Part model, mm, in its own coordinate system. Face numbers are marked on the shaded views. A direction names the side the tool comes from. Round coordinates to 2 decimals unless told otherwise and drop trailing zeros. Loops run counter-clockwise (first coordinate to the right, second up) from the corner with the lowest first, then second, coordinate; pieces in that order, holes last. Notation, with made-up numbers: (50.25, -19.75) -> (78.25, -19.75) arc R25 cw to (78.25, 4.25) -> close; hole circle Ø9 at (45.5, -35.75). An arc over 180 degrees is marked (long way). Answer as CSV lines item,"result".
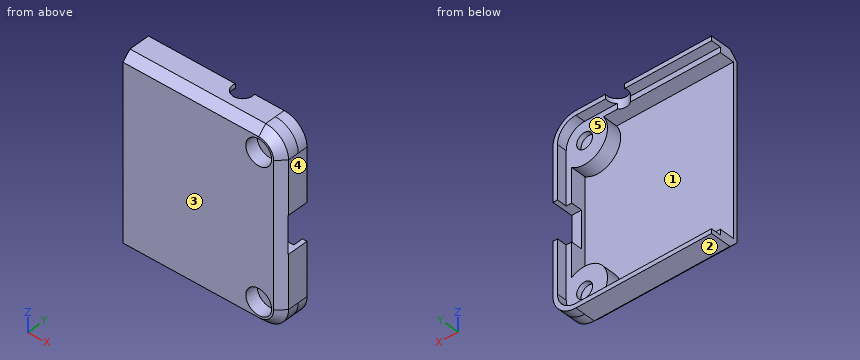
from build123d import *

# Parameters (mm, degrees)
CYLINDER003_R     = 2
CYLINDER003_DEPTH = 10
CYLINDER001_R     = 2
CYLINDER001_DEPTH = 10
SKETCH037_W       = 7.5
SKETCH037_H       = 7.5
EXTRUDE045_DEPTH  = 10
SKETCH032_R       = 2.6
EXTRUDE043_DEPTH  = 0.8
EXTRUDE050_DEPTH  = 3
EXTRUDE051_DEPTH  = 0.8
EXTRUDE038_DEPTH  = 2


with BuildPart() as shutter_cable001:
    # Cylinder003 → Cylinder003 (new body)
    with BuildSketch(Plane(origin=(19.5, 0, 24.5), x_dir=(1, 0, 0), z_dir=(0, 0, 1))):
        Circle(CYLINDER003_R)
    extrude(amount=CYLINDER003_DEPTH)


with BuildPart() as battery_cable:
    # Cylinder001 → Cylinder001 (new body)
    with BuildSketch(Plane(origin=(-70.5, 0, 12), x_dir=(0, 0, 1), z_dir=(-1, 0, 0))):
        Circle(CYLINDER001_R)
    extrude(amount=CYLINDER001_DEPTH)


with BuildPart() as common_sub:
    # Sketch037 → Extrude045 (new body)
    with BuildSketch(Plane.YZ.offset(35)):
        with Locations((0, 12)):
            Rectangle(SKETCH037_W, SKETCH037_H)
    extrude(amount=EXTRUDE045_DEPTH)


with BuildPart() as common_sub_1:
    # Extrude045 placement: moved
    add(common_sub.part.moved(Location((-9.5, 0, 0))))

    # Fusion033: union shutter cable001, battery cable
    add(shutter_cable001.part)
    add(battery_cable.part)


with BuildPart() as sweep_body:
    # Sweep: sweep along a path in Sketch034
    with BuildLine(Plane.XZ.offset(10)) as sweep_path:
        Line((32, 12), (32, 26.4))
        ThreePointArc((32, 26.4), (30.652691, 29.652691), (27.4, 31))
        Line((27.4, 31), (-39.9, 31))
    # Sketch033 → Sweep (sweep)
    with BuildSketch(Plane.YZ):
        Polygon((-5.3, 29.4), (-3.7, 31), (-3.7, 32), (-6, 32), (-6, 29.4), align=None)
    sweep(path=sweep_path.line)


with BuildPart() as fusion:
    # Sketch032 → Extrude043 (new body)
    with BuildSketch(Plane.XZ.offset(10)):
        with Locations((27.4, 26.4)):
            Circle(SKETCH032_R)
    extrude(amount=EXTRUDE043_DEPTH)


with BuildPart() as fusion_1:
    # Extrude043 placement: moved
    add(fusion.part.moved(Location((0, 5.5, 0))))

    # Fusion: union Sweep body
    add(sweep_body.part)


with BuildPart() as screw_hole_bottom002:
    # Sketch003 → Revolve (revolve)
    with BuildSketch(Plane.XY):
        Polygon((1.6, 3), (1.6, 2), (0, 2), (0, 1.8), (2.6, 1.8), (2.6, 0), (4.6, 0), (4.6, 3), align=None)
    revolve(axis=Axis((0, 0, 0), (0, 1, 0)))


with BuildPart() as screw_hole_bottom002_1:
    # Body003 placement: moved
    add(screw_hole_bottom002.part.moved(Location((27.4, -4.5, 26.4))))


with BuildPart() as bottom009:
    # Sketch041 → Extrude050 (new body)
    with BuildSketch(Plane.XZ.offset(10)):
        with BuildLine():
            ThreePointArc((32, 26.4), (30.652691, 29.652691), (27.4, 31))
            Line((27.4, 31), (0.1, 31))
            Line((0.1, 31), (0.1, 29))
            Line((0.1, 29), (27.4, 29))
            ThreePointArc((30, 26.4), (29.238478, 28.238478), (27.4, 29))
            Line((30, 12), (30, 26.4))
            Line((32, 12), (30, 12))
            Line((32, 26.4), (32, 12))
        make_face()
    extrude(amount=EXTRUDE050_DEPTH)


with BuildPart() as bottom009_1:
    # Extrude050 placement: moved
    add(bottom009.part.moved(Location((0, 8.5, 0))))


with BuildPart() as bottom010:
    # Sketch042 → Extrude051 (new body)
    with BuildSketch(Plane.XZ.offset(10)):
        with BuildLine():
            ThreePointArc((32, 26.4), (30.652691, 29.652691), (27.4, 31))
            Line((27.4, 31), (0.1, 31))
            Line((0.1, 31), (0.1, 12))
            Line((0.1, 12), (32, 12))
            Line((32, 26.4), (32, 12))
        make_face()
    extrude(amount=EXTRUDE051_DEPTH)


with BuildPart() as bottom010_1:
    # Extrude051 placement: moved
    add(bottom010.part.moved(Location((0, 5.5, 0))))


with BuildPart() as bottom:
    # Sketch030 → Extrude038 (new body)
    with BuildSketch(Plane.XZ.offset(10)):
        with BuildLine():
            ThreePointArc((32, 26.4), (30.652691, 29.652691), (27.4, 31))
            Line((27.4, 31), (0.1, 31))
            Line((0.1, 31), (0.1, 30.1))
            Line((0.1, 30.1), (27.4, 30.1))
            ThreePointArc((31.1, 26.4), (30.016295, 29.016295), (27.4, 30.1))
            Line((31.1, 12), (31.1, 26.4))
            Line((32, 12), (31.1, 12))
            Line((32, 26.4), (32, 12))
        make_face()
    extrude(amount=EXTRUDE038_DEPTH)


with BuildPart() as bottom_1:
    # Extrude038 placement: moved
    add(bottom.part.moved(Location((0, 10.5, 0))))

    # Fusion029: union screw hole bottom002, bottom009, bottom010
    add(screw_hole_bottom002_1.part)
    add(bottom009_1.part)
    add(bottom010_1.part)

    # Cut: cut Fusion
    add(fusion_1.part, mode=Mode.SUBTRACT)


with BuildPart() as part_mirroring004:
    # Part__Mirroring004: instance of bottom
    add(bottom_1.part.mirror(Plane(origin=(0, 0, 12), x_dir=(0, 1, 0), z_dir=(0, 0, 1))))


with BuildPart() as bottom007:
    # Fusion031 base: copy of bottom
    add(bottom_1.part)

    # Fusion031: union Part__Mirroring004
    add(part_mirroring004.part)

    # Cut026: cut common sub
    add(common_sub_1.part, mode=Mode.SUBTRACT)


solid = bottom007.part
Q1. Drill centre lines: line 1 along Z through (x, y) = (3, -0.9); line 2 along Z through (x, y) = (27.4, -3.75); line 3 along Z through (x, y) = (11, -3.55). Where is each one in solid material? Low to high.
Geometry results:
line 1,"-7 to -6.1, 30.1 to 31"
line 2,"-6.95 to -5, 0.2 to 2.2, 21.8 to 23.8, 29 to 30.95"
line 3,"-7 to -5, 29 to 31"
Q2. Drop flat-ended pins along their axis: P1, Ø0.9, axis at y = -3.5, z = 11.5, coming from the -X side; P2, Ø2, axis at y = 0, z = 22, coming from the -X side; P3, Ø2, axis at x = 21, z = 19.5, coming from the +Y side; P4, Ø3, axis at x = 16.5, y = -4.5, coming from the +Z side. Give the stop position or say it passes through.
Geometry results:
P1,"x = 30"
P2,"x = 31.1"
P3,"y = -4.5"
P4,"z = 31"
Q3. Saw through at D-D, the plane z = 25.5. Write the cut outline in (x, y), then the cut area to 3 significant figures.
Geometry results:
outline,"(0.1, -5.3) -> (24.96, -5.3) -> (24.96, -2.7) -> (29.84, -2.7) -> (29.84, -5.3) -> (30.4, -5.3) -> (32, -3.7) -> (32, 0.5) -> (31.1, 0.5) -> (31.1, -1.5) -> (28.72, -1.5) -> (28.72, -2.5) -> (26.08, -2.5) -> (26.08, -1.5) -> (22.89, -1.5) -> (22.89, -4.5) -> (0.1, -4.5) -> close"
area,"38.0 mm2"
Q4. Which spindle directions (+Z, -Z, +X, -X, +Y, -Y) get a long thin tool onto all of the face, cutting with end or side? Do the marked faces 4 and 5. Say none if no direction does.
Geometry results:
face 4,"+Z, -Z, +X, +Y, -Y"
face 5,"-X, +Y"
Q5. Saw through at C-C, the plane x = 14. Write the cut outline in (y, z).
Geometry results:
outline,"(-5.3, -5.4) -> (-3.7, -7) -> (0.5, -7) -> (0.5, -6.1) -> (-1.5, -6.1) -> (-1.5, -5) -> (-4.5, -5) -> (-4.5, 29) -> (-1.5, 29) -> (-1.5, 30.1) -> (0.5, 30.1) -> (0.5, 31) -> (-3.7, 31) -> (-5.3, 29.4) -> close"
Q6. Two-plate mould, pull along Z, no slides. Class the marked faces 1, 2 and 3: pulls with the +Z half, pulls with the -Z half, needs draft (parallel to the pull), parting line crosses it, or undercut.
Geometry results:
face 1,"undercut"
face 2,"pulls with the -Z half"
face 3,"needs draft"
Q7. Saw through at A-A, the plane y = -3.1. Write the cut outline in (x, z).
Geometry results:
outline,"(0.1, -7) -> (27.4, -7) arc R4.6 ccw to (32, -2.4) -> (32, 8.25) -> (30, 8.25) -> (30, 1.39) arc R4.6 ccw to (23.61, -5) -> (0.1, -5) -> close; (0.1, 29) -> (23.61, 29) arc R4.6 ccw to (30, 22.61) -> (30, 15.75) -> (32, 15.75) -> (32, 26.4) arc R4.6 ccw to (27.4, 31) -> (0.1, 31) -> close; hole circle Ø5.2 at (27.4, -2.4); hole circle Ø5.2 at (27.4, 26.4)"
Q8. Saw through at B-B, the plane y = 0. Write the cut outline in (x, z).
Geometry results:
outline,"(0.1, -7) -> (27.4, -7) arc R4.6 ccw to (32, -2.4) -> (32, 8.25) -> (31.1, 8.25) -> (31.1, -2.4) arc R3.7 cw to (27.4, -6.1) -> (0.1, -6.1) -> close; (0.1, 30.1) -> (17.5, 30.1) -> (17.5, 31) -> (0.1, 31) -> close; (21.5, 30.1) -> (27.4, 30.1) arc R3.7 cw to (31.1, 26.4) -> (31.1, 15.75) -> (32, 15.75) -> (32, 26.4) arc R4.6 ccw to (27.4, 31) -> (21.5, 31) -> close"
